Here's how the part is built. I have some questions about the finished solid (model axes, mm). A direction names the side the tool comes from. Coordinates: 2 decimals unless noted, no trailing zeros. Order: outer loops, then holes, each group sorted by start corner. A loop starts at its lowest first (then second) coordinate and runs counter-clockwise, first axis right, second up. Notation, with made-up numbers: M 9,81 L 28,81 A11 cw 28,90 Z; hole C 20.25,-4 d9. An arc over 180 degrees is marked long. One line per question, with ' | ' between items. Start each with the question number.
Autodesk Inventor part; units mm, degrees
ref_plane "YZ Plane" through (0, 0, 0) normal (1, 0, 0) x (0, 1, 0)
ref_plane "XZ Plane" through (0, 0, 0) normal (0, 1, 0) x (-1, 0, 0)
ref_plane "XY Plane" through (0, 0, 0) normal (0, 0, 1) x (1, 0, 0)
sketch "Sketch1" plane through (0, 0, 0) normal (0, 1, 0) x (-1, 0, 0)
  line L0 (5.5, 19.825) -> (-5.5, 19.825)
  line L1 (-8.5, 16.825) -> (-8.5, -16.825)
  line L2 (-5.5, -19.825) -> (5.5, -19.825)
  line L3 (8.5, -16.825) -> (8.5, 16.825)
  line L4 (8.5, 19.825) -> (-8.5, -19.825) construction
  line L5 (-8.5, 19.825) -> (8.5, -19.825) construction
  line L6 (-5.5, 19.825) -> (-8.5, 16.825)
  line L7 (5.5, 19.825) -> (8.5, 16.825)
  line L8 (8.5, -16.825) -> (5.5, -19.825)
  line L9 (-5.5, -19.825) -> (-8.5, -16.825)
  circle A0 centre (3.9654, 16.6011) radius 0.5
  circle A1 centre (3.9654, 14.0611) radius 0.5
  circle A2 centre (3.9654, 11.5211) radius 0.5
  circle A3 centre (3.9654, 6.4411) radius 0.5
  circle A4 centre (3.9654, 3.9011) radius 0.5
  circle A5 centre (3.9654, 1.3611) radius 0.5
  circle A6 centre (3.9654, -1.1789) radius 0.5
  line L10 (4.9485, 17.9314) -> (2.9084, 17.9314)
  line L11 (2.9084, 17.9314) -> (2.9084, -2.5092)
  line L12 (2.9084, -2.5092) -> (4.9485, -2.5092)
  line L13 (4.9485, -2.5092) -> (4.9485, 17.9314)
  circle A7 centre (2.8556, -8.4694) radius 1.5
  circle A8 centre (-5.4926, 10.8475) radius 0.5
  circle A9 centre (-5.4926, 8.3075) radius 0.5
  circle A10 centre (-5.4926, 5.7675) radius 0.5
  circle A11 centre (-5.4926, 3.2275) radius 0.5
  circle A12 centre (-5.4926, -1.9498) radius 0.5
  circle A13 centre (-5.4926, -4.4898) radius 0.5
  circle A14 centre (-5.4926, -7.0298) radius 0.5
  circle A15 centre (-5.4926, -9.5698) radius 0.5
  circle A16 centre (-5.5, -12.1098) radius 0.5
  circle A17 centre (0, -16.105) radius 1.5
  circle A18 centre (0, 17.225) radius 1.5
  circle A19 centre (3.9285, 8.9811) radius 0.5
  point P0 (0, 0)
  dimension "d0" = 17
  dimension "d1" = 39.65
  dimension "d2" = 3
  dimension "d3" = 3
  dimension "d4" = 3
  dimension "d5" = 3
  dimension "d6" = 3
  dimension "d7" = 3
  dimension "d8" = 3
  dimension "d9" = 3
  dimension "d10" = 1
  dimension "d11" = 1
  dimension "d12" = 1
  dimension "d13" = 1
  dimension "d14" = 1
  dimension "d15" = 1
  dimension "d16" = 1
  dimension "d17" = 2.54
  dimension "d18" = 2.54
  dimension "d19" = 2.54
  dimension "d20" = 2.54
  dimension "d21" = 2.54
  dimension "d23" = 3
  dimension "d24" = 1
  dimension "d25" = 1
  dimension "d26" = 1
  dimension "d27" = 1
  dimension "d28" = 2.54
  dimension "d29" = 2.54
  dimension "d30" = 2.54
  dimension "d31" = 1
  dimension "d32" = 1
  dimension "d33" = 1
  dimension "d34" = 1
  dimension "d35" = 2.54
  dimension "d36" = 2.54
  dimension "d37" = 2.54
  dimension "d39" = 2.54
  dimension "d51" = 3
  dimension "d52" = 3
  dimension "d53" = 2.6
  dimension "d54" = 3.72
  dimension "d59" = 33.33
  dimension "d60" = 1
  dimension "d61" = 2.54
  dimension "d62" = 2.54
  dimension "d63" = 1.3303
  dimension "d64" = 1.3303
extrude "Extrusion2" add sketch "Sketch1" along normal blind 8.4 contours L13 L12 L11 L10 | A19
extrude "Extrusion3" add sketch "Sketch1" along normal blind 5 contours A7
extrude "Extrusion4" cut sketch "Sketch1" along normal blind 1.7 contours L7 L3 L8 L2 L9 L1 L6 L0 | A17 | A18
extrude "Extrusion5" add sketch "Sketch1" along normal blind 1.7 contours L7 L3 L8 L2 L9 L1 L6 L0 | A17 | A18
fillet "Fillet1" radius 1 1 edges at (-1.3556, 5, -8.4694)
sketch "Sketch2" plane through (0, 1.7, 0) normal (0, 1, 0) x (1, 0, 0)
  line L0 (-0.041, -10.2921) -> (-0.041, 12.3756) construction
  line L1 (-0.041, 12.3756) -> (3.5412, 12.3756) construction
  line L2 (3.5412, 12.3756) -> (3.5412, -10.2921) construction
  line L3 (3.5412, -10.2921) -> (-0.041, -10.2921) construction
  point P0 (0, 0)
extrude "Extrusion6" cut sketch "Sketch1" against normal blind 10 contours A17 | A18
extrude "Extrusion7" cut sketch "Sketch1" along normal through all contours A17 | A18
extrude "Extrusion8" cut sketch "Sketch1" along normal up to next contours A19
equation "\"d3\" = d2"
equation "\"d4\" = d2"
equation "\"d5\" = d4"
equation "\"d6\" = d2"
equation "\"d7\" = d6"
equation "\"d8\" = d2"
equation "\"d9\" = d8"
properties part number "Driver TPA"
1. We'd pull the mould along X, two halves only. Please class faces 3 (the face through (-3.86, 4.14, 17.09)), 4 (the face through (-4, 5, 17.931)), 5 (the face through (-1.75, 2.834, -9.483)): released by +X, released by -X, zero draft, split by the parting line, or undercut.
2. Will these pins go through, and if not, where does the flat tip stop? pin 1 (3 mm diameter, centred on y = 4, z = -1.5, fed in from +X); pin 2 (1 mm diameter, centred on x = -4, y = 6, fed in from +Z); pin 3 (1 mm diameter, centred on x = -4, y = 6, fed in from -Z).
3. I need wall thicknesses on line 1 (Z direction, x = 0, y = 0.9) (3 decimals); line 2 (Z direction, x = -4.75, y = 4); line 3 (Y direction, x = 6.75, z = 11). Which ranges of each line are inside material? Lowest first, please.
4. Imagine slicing it at A-A (x = 0). List the corners of the cut face in (y, z) for me (3 decimals), then the cut area to 3 significant figures.
5. Imagine slicing it at D-D (x = 4.25). List the corners of the cut face in (y, z) for me (3 decimals).
6. Which directions (+Z, -Z, +X, -X, +Y, -Y) give clear straight access to the entire face, cutting with the end or side of a thin tool? Please do faces 1 (the face through (-3.466, 4.141, -1.201)), 2 (the face through (-2.908, 5, 8)).
7. Imagine slicing it at C-C (z = 0). List the corners of the cut face in (x, y) for me.
8. Imagine slicing it at B-B (y = 2.75). Count the separate pieces of the cut face and the enclosed holes in it, then the cut area to 3 significant figures.
Entries:
1) face 3: undercut | face 4: zero draft | face 5: split by the parting line
2) pin 1: x = -2.91 | pin 2: z = 17.93 | pin 3: z = -2.51
3) line 1: -19.825 to -17.605, -14.605 to 15.725, 18.725 to 19.825 | line 2: -2.51 to 17.93 | line 3: 0 to 1.7
4) outline: M 0,-19.825 L 1.7,-19.825 L 1.7,-17.605 L 0,-17.605 Z; M 0,-14.605 L 1.7,-14.605 L 1.7,15.725 L 0,15.725 Z; M 0,18.725 L 1.7,18.725 L 1.7,19.825 L 0,19.825 Z | area: 57.2 mm²
5) outline: M 0,-19.825 L 1.7,-19.825 L 1.7,19.825 L 0,19.825 Z
6) face 1: +Y, -Y | face 2: +Z, +X, +Y
7) outline: M -8.5,0 L 8.5,0 L 8.5,1.7 L -2.91,1.7 L -2.91,8.4 L -4.95,8.4 L -4.95,1.7 L -8.5,1.7 Z
8) separate pieces: 2 | enclosed holes: 8 | area: 42.5 mm²
